```python
from build123d import *

# Parameters (mm, degrees)
SKETCH1_R           = 6.35
BOSS_EXTRUDE1_DEPTH = 44.45
CHAMFER1_SIZE       = 0.254


with BuildPart() as part:
    # Sketch1 → Boss-Extrude1 (new body)
    with BuildSketch(Plane(origin=(0, 0, 0), x_dir=(1, 0, 0), z_dir=(0, 1, 0))):
        with Locations(Location((0, 0, 0), (0, 0, 270))):
            Circle(SKETCH1_R)
    extrude(amount=BOSS_EXTRUDE1_DEPTH)

    # Sketch3 → 1/4-20 Tapped Hole1 (revolve, cut)
    with BuildSketch(Plane(origin=(0, 44.45, 0), x_dir=(0, 0, 1), z_dir=(1, 0, 0))):
        Polygon((0, 0), (0, 44.45), (3.81, 44.45), (2.5527, 43.1927), (2.5527, 1.2573), (3.81, 0), align=None)
    revolve(axis=Axis((0, 50.8, 0), (0, -1, 0)), mode=Mode.SUBTRACT)

    # Chamfer1
    chamfer1_edges = [part.edges().sort_by_distance(p)[0] for p in [
        (0, 0, -6.35),
        (0, 44.45, -6.35),
    ]]
    chamfer(chamfer1_edges, length=CHAMFER1_SIZE)


solid = part.part
```
CAD build for the part. Positions are in the model's coordinates, mm. Round coordinates to 2 decimals unless told otherwise and drop trailing zeros. Write each loop counter-clockwise with the first axis right and the second up, starting at its lowest first coordinate (ties: lowest second). Pieces come first, ordered by that corner, then holes. Notation, with made-up numbers: (-5.5, -15) - (43.5, -15) arc R10 cw to (43.5, -10) - close; hole circle Ø8 at (-31, 62.25). An arc over 180 degrees is marked (long way). Return JSON: item names as keys, results as strings. Group by question number.
Item 1: Band-saw the part on A-A on x = 0. List the corners of the cut face in (y, z).
Item 2: Flat gauge pins, fed straight in: pin 1 Ø1 at (y, z) = (18, 3.5) entering from -X; pin 2 Ø3 at (x, y) = (2.5, 13.5) entering from -Z. Where does each tip first touch, or does it go through?
Item 3: Band-saw the part on B-B on z = 0. List the corners of the cut face in (x, y).
Item 4: Probe probe 1 along X at (y, z) = (41.5, 0); probe 2 along X at (y, z) = (42, -0.75); probe 3 along Z at (x, y) = (0.5, 9.5). List the from-to ranges inside material, lowest first.
Item 5: Band-saw the part on C-C on y = 34. List the corners of the cut face in (x, z).
Item 6: Mould opens along Z. For faces 1 (the face through (-3.86, 21.92, -5.04)), 2 (the face through (-0.767, 22.519, 2.435)), 3 (the face through (3, 0, 3)) say: +Z half, -Z half, draft (parallel to the pull), parting line (faces both ways), or undercut.
Resolved:
{
 "1": {"outline": "(0, -6.1) - (0.25, -6.35) - (44.2, -6.35) - (44.45, -6.1) - (44.45, -3.81) - (43.19, -2.55) - (1.26, -2.55) - (0, -3.81) - close; (0, 3.81) - (1.26, 2.55) - (43.19, 2.55) - (44.45, 3.81) - (44.45, 6.1) - (44.2, 6.35) - (0.25, 6.35) - (0, 6.1) - close"},
 "2": {"pin 1": "stops at x = -5.6", "pin 2": "stops at z = -6.27"},
 "3": {"outline": "(-6.35, 0.25) - (-6.1, 0) - (-3.81, 0) - (-2.55, 1.26) - (-2.55, 43.19) - (-3.81, 44.45) - (-6.1, 44.45) - (-6.35, 44.2) - close; (2.55, 1.26) - (3.81, 0) - (6.1, 0) - (6.35, 0.25) - (6.35, 44.2) - (6.1, 44.45) - (3.81, 44.45) - (2.55, 43.19) - close"},
 "4": {"probe 1": "x = -6.35 to -2.55, 2.55 to 6.35", "probe 2": "x = -6.31 to -2.44, 2.44 to 6.31", "probe 3": "z = -6.33 to -2.5, 2.5 to 6.33"},
 "5": {"outline": "circle Ø12.7 at (0, 0); hole circle Ø5.11 at (0, 0)"},
 "6": {"face 1": "parting line", "face 2": "undercut", "face 3": "draft"}
}
